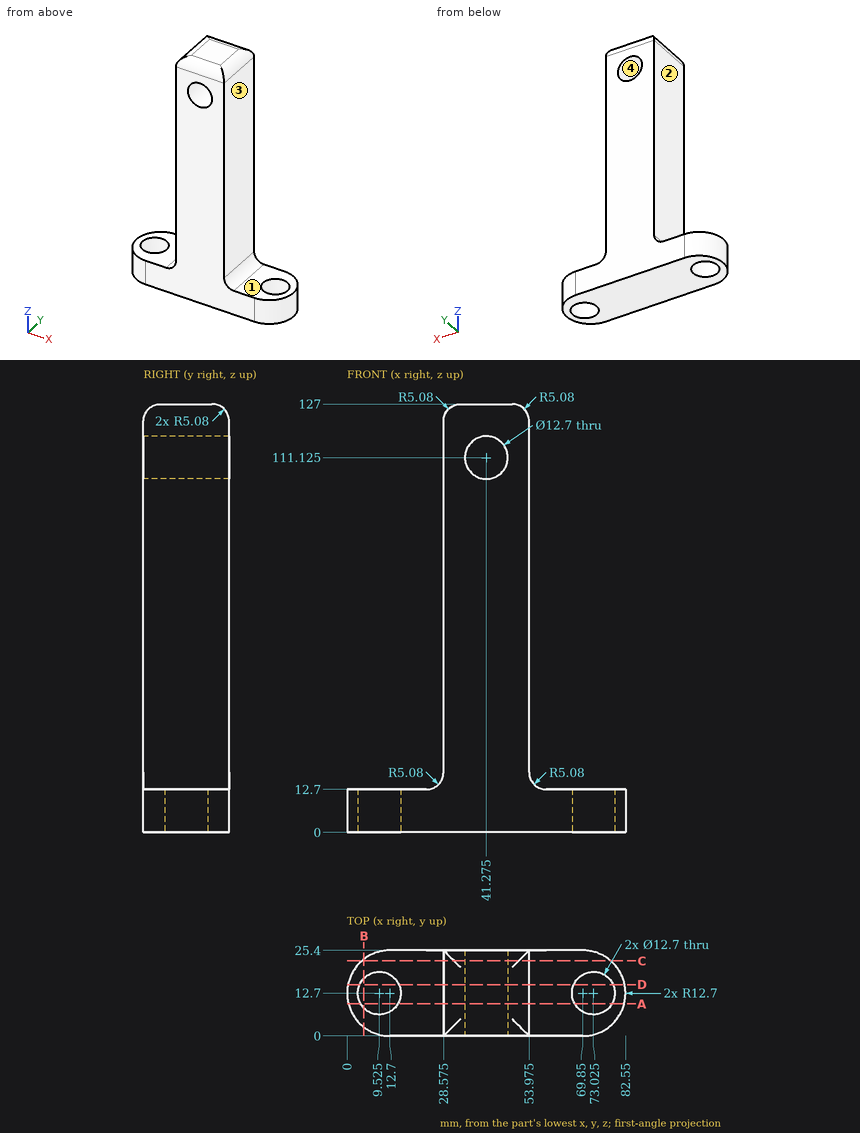
Print and shaded views of the part. All mm, measured from the part's lowest x, y and z. Round coordinates to 2 decimals unless told otherwise and drop trailing zeros. Write each loop counter-clockwise with the first axis right and the second up, starting at its lowest first coordinate (ties: lowest second). Pieces come first, ordered by that corner, then holes.
Item 1: Two-plate mould, pull along X, no slides. Class the marked faces 1, 2, 3 and 4: +X half, -X half, draft (parallel to the pull), parting line (faces both ways), or undercut.
Results:
face 1: draft
face 2: -X half
face 3: +X half
face 4: undercut
Item 2: Cut at C-C, the plane y = 22.25. Give the cut face in (x, z) (3 decimals), plus the area to 3 significant figures.
Results:
outline: (4.328, 0) - (78.222, 0) - (78.222, 12.7) - (59.055, 12.7) arc R5.08 cw to (53.975, 17.78) - (53.975, 121.92) arc R5.08 ccw to (50.825, 126.619) - (31.725, 126.619) arc R5.08 ccw to (28.575, 121.92) - (28.575, 17.78) arc R5.08 cw to (23.495, 12.7) - (4.328, 12.7) - close; hole circle Ø12.7 at (41.275, 111.125)
area: 3,710 mm2
Item 3: Drop flat-ended pins along their axis: pin 1 Ø8 at (x, y) = (14, 20) entering from +Z; pin 2 Ø12.5 at (y, z) = (14, 91.5) entering from -X (3 decimals); pin 3 Ø11.5 at (x, z) = (41.275, 111.125) entering from +Y; pin 4 Ø12.5 at (y, z) = (13, 83) entering from +X (3 decimals). Give the stop position or say it passes through.
Results:
pin 1: stops at z = 12.7
pin 2: stops at x = 28.575
pin 3: passes through
pin 4: stops at x = 53.975
Item 4: Cut at D-D, the plane y = 15.25. Count the separate pieces of the cut face and the enclosed holes in it, plus the area to 3 significant figures.
Results:
separate pieces: 3
enclosed holes: 1
area: 3,520 mm2
Item 5: Probe L1, parallel to X at y = 16.25, z = 110.5 (3 decimals); L2, parallel to X at y = 18.5, z = 10; L3, parallel to X at y = 11, z = 120 (3 decimals). List the from-to ranges inside material, lowest first.
Results:
L1: x = 28.575 to 34.956, 47.594 to 53.975
L2: x = 1.4 to 6.94, 12.11 to 70.44, 75.61 to 81.15
L3: x = 28.575 to 53.975
Item 6: Cut at A-A, the plane y = 9.5. Give the cut face in (x, z) (3 decimals).
Results:
outline: (0.41, 0) - (4.04, 0) - (4.04, 12.7) - (0.41, 12.7) - close; (15.01, 0) - (67.54, 0) - (67.54, 12.7) - (59.055, 12.7) arc R5.08 cw to (53.975, 17.78) - (53.975, 121.92) arc R5.08 ccw to (48.895, 127) - (33.655, 127) arc R5.08 ccw to (28.575, 121.92) - (28.575, 17.78) arc R5.08 cw to (23.495, 12.7) - (15.01, 12.7) - close; (78.51, 0) - (82.14, 0) - (82.14, 12.7) - (78.51, 12.7) - close; hole circle Ø12.7 at (41.275, 111.125)
Item 7: Cut at B-B, the plane x = 5. Give the cut face in (y, z), plus the area to 3 significant figures.
Results:
outline: (2.6, 0) - (8.25, 0) - (8.25, 12.7) - (2.6, 12.7) - close; (17.15, 0) - (22.8, 0) - (22.8, 12.7) - (17.15, 12.7) - close
area: 143 mm2
